Read the model definition and answer for the solid it produces. Units are mm, in the model's axes. A direction names the side the tool comes from. Coordinates: 2 decimals unless noted, no trailing zeros. Loops run counter-clockwise (first coordinate to the right, second up) from the corner with the lowest first, then second, coordinate; pieces in that order, holes last. Notation, with made-up numbers: (-27, 26.25) - (-9, 26.25) arc R35 ccw to (-9, 58.25) - close; hole circle Ø5 at (72.25, -33.75). An arc over 180 degrees is marked (long way). Use CSV: the item, a comma, the result in double quotes.
Autodesk Inventor part; units mm, degrees
ref_plane "Work Plane1" through (12.7, 70.5404, -12.7) normal (0, 0, -1) x (-1, 0, 0)
ref_plane "YZ Plane" through (0, 0, 0) normal (1, 0, 0) x (0, 1, 0)
ref_plane "XZ Plane" through (0, 0, 0) normal (0, 1, 0) x (-1, 0, 0)
sketch "Sketch1" plane through (0, 0, 0) normal (1, 0, 0) x (0, 1, 0)
  line L0 (0, 0) -> (76.2, 0)
  line L1 (76.2, 0) -> (76.2, -114.3)
  line L2 (76.2, -114.3) -> (0, -114.3)
  line L3 (0, -114.3) -> (0, 0)
  dimension "d0" = 76.2
  dimension "d1" = 114.3
extrude "Extrusion1" add sketch "Sketch1" along normal blind 12.7
sketch "Sketch2" plane through (12.7, 0, 0) normal (1, 0, 0) x (0, 0, -1)
  line L0 (0, 76.2) -> (0, 0)
  line L1 (0, 76.2) -> (25.4, 76.2)
  line L2 (25.4, 76.2) -> (25.4, 70.5404)
  line L3 (25.4, 70.5404) -> (0, 70.5404)
  line L4 (0, 70.5404) -> (0, 76.2)
  dimension "d4" = 25.4
extrude "Extrusion2" add sketch "Sketch2" along normal blind 12.7
sketch "Sketch3" plane through (0, 76.2, 0) normal (0, 1, 0) x (1, 0, 0)
  line L0 (0, 0) -> (0, 114.3)
  line L1 (0, 0) -> (25.4, 0)
  line L2 (25.4, 25.4) -> (25.4, 0)
  line L3 (12.7, 25.4) -> (25.4, 25.4)
  line L4 (12.7, 114.3) -> (12.7, 25.4)
  line L5 (0, 114.3) -> (12.7, 114.3)
  line L6 (12.7, 25.4) -> (25.4, 25.4)
  line L7 (22.225, 25.4) -> (22.225, 0)
  line L8 (0, 0) -> (25.4, 0)
  dimension "d8" = 3.175
extrude "Extrusion3" add sketch "Sketch3" along normal blind 25.4 contours L7 L3 L2 L1
sketch "Sketch4" plane through (0, 0, 0) normal (0, 0, 1) x (1, 0, 0)
  line L0 (0, 76.2) -> (22.225, 76.2)
  line L1 (0, 76.2) -> (22.225, 101.6)
  line L2 (22.225, 101.6) -> (19.8356, 103.6908)
  line L3 (19.8356, 103.6908) -> (0, 81.0215)
  line L4 (22.225, 101.6) -> (25.4, 101.6)
  line L5 (22.225, 76.2) -> (22.225, 101.6)
  line L6 (0, 76.2) -> (0, 81.0215)
  line L7 (22.225, 97.3812) -> (20.1342, 99.2106)
  line L8 (3.175, 76.2) -> (3.175, 79.8286)
  point P0 (0, 0)
  dimension "d11" = 3.175
  dimension "d12" = 3.175
  dimension "d13" = 3.175
extrude "Extrusion4" add sketch "Sketch4" against normal blind 3.175 contours L1 L8 L0 | L6 L3 L2 L1 | L1 L5 L7
ref_plane "Work Plane1" through (12.7, 70.5404, -12.7) normal (0, 0, -1) x (-1, 0, 0)
mirror "Mirror1" about plane through (12.7, 70.5404, -12.7) normal (0, 0, -1) of "Extrusion4"
sketch "Sketch5" plane through (25.4, 0, 0) normal (1, 0, 0) x (0, 0, -1)
  line L0 (0, 70.5404) -> (0, 101.6)
  line L1 (0, 70.5404) -> (25.4, 70.5404)
  line L2 (25.4, 70.5404) -> (25.4, 101.6)
  line L3 (0, 101.6) -> (25.4, 101.6)
  circle A0 centre (12.7, 88.9) radius 6.35
  line L4 (0, 76.2) -> (25.4, 76.2)
  circle A1 centre (12.7, 98.425) radius 1.778
  point P0 (0, 0)
  dimension "d16" = 12.7
  dimension "d17" = 25.4
  dimension "d18" = 25.4
  dimension "d19" = 12.7
  dimension "d20" = 12.7
  dimension "d21" = 3.556
  dimension "d22" = 9.525
extrude "Extrusion5" cut sketch "Sketch5" against normal blind 3.175 contours A1
pattern_circular "Circular Pattern1" count 8 over 360 about axis through (25.4, 88.9, -12.7) along (1, 0, 0) of "Extrusion5"
sketch "Sketch6" plane through (0, 0, 0) normal (-1, 0, 0) x (0, 0, 1)
  line L0 (0, 0) -> (-114.3, 0)
  line L1 (-20.0153, 0) -> (-20.0153, 59.8716) construction
  line L2 (-10.4903, 0) -> (-10.4903, 59.8716)
  line L3 (-29.5403, 59.8716) -> (-29.5403, 0)
  arc A0 (-29.5403, 0) -> (-10.4903, 0) centre (-20.0153, 0) ccw
  arc A1 (-10.4903, 59.8716) -> (-29.5403, 59.8716) centre (-20.0153, 59.8716) ccw
  line L4 (-20.0153, 59.8716) -> (-96.2153, 59.8716) construction
  line L5 (-20.0153, 69.3966) -> (-96.2153, 69.3966)
  line L6 (-96.2153, 50.3466) -> (-20.0153, 50.3466)
  arc A2 (-20.0153, 50.3466) -> (-20.0153, 69.3966) centre (-20.0153, 59.8716) ccw
  arc A3 (-96.2153, 69.3966) -> (-96.2153, 50.3466) centre (-96.2153, 59.8716) ccw
  line L7 (-96.2153, 59.8716) -> (-96.2153, 0) construction
  line L8 (-105.7403, 59.8716) -> (-105.7403, 0)
  line L9 (-86.6903, 0) -> (-86.6903, 59.8716)
  arc A4 (-86.6903, 59.8716) -> (-105.7403, 59.8716) centre (-96.2153, 59.8716) ccw
  arc A5 (-105.7403, 0) -> (-86.6903, 0) centre (-96.2153, 0) ccw
  line L10 (-114.3, 0) -> (-114.3, 76.2)
  line L11 (0, 0) -> (0, 81.0215)
  point P0 (-20.0153, 29.9358)
  point P1 (-58.1153, 59.8716)
  point P2 (-96.2153, 29.9358)
  dimension "d28" = 19.05
  dimension "d29" = 76.2
  dimension "d30" = 19.05
  dimension "d31" = 19.05
  dimension "d32" = 95.25
  dimension "d36" = 116.2307
  dimension "d37" = 10.4903
sketch "Sketch7" plane through (12.7, 0, 0) normal (1, 0, 0) x (0, 0, -1)
  line L0 (25.4, 70.5404) -> (0, 70.5404)
  line L1 (0, 70.5404) -> (0, 0)
  line L2 (0, 0) -> (114.3, 0) construction
  line L3 (114.3, 0) -> (114.3, 76.2)
  line L4 (114.3, 76.2) -> (25.4, 76.2)
  line L5 (25.4, 76.2) -> (25.4, 70.5404)
  line L6 (105.7403, 59.8716) -> (105.7403, 0)
  line L7 (20.0153, 69.3966) -> (96.2153, 69.3966)
  line L8 (0, 0) -> (0, 81.0215)
  line L9 (0, 81.0215) -> (3.175, 81.0215)
  line L10 (3.175, 76.2) -> (3.175, 81.0215)
  line L11 (3.175, 76.2) -> (22.225, 76.2)
  line L12 (22.225, 76.2) -> (22.225, 81.0215)
  line L13 (25.4, 81.0215) -> (22.225, 81.0215)
  line L14 (25.4, 81.0215) -> (25.4, 76.2)
  line L15 (25.4, 76.2) -> (114.3, 76.2)
  line L16 (114.3, 76.2) -> (114.3, 0)
  line L17 (114.3, 0) -> (0, 0)
  arc A0 (105.7403, 59.8716) -> (86.6903, 59.8716) centre (96.2153, 59.8716) ccw
  arc A1 (96.2153, 50.3466) -> (96.2153, 69.3966) centre (96.2153, 59.8716) ccw
  line L18 (96.2153, 50.3466) -> (20.0153, 50.3466)
  line L19 (86.6903, 0) -> (86.6903, 59.8716)
  arc A2 (86.6903, 0) -> (105.7403, 0) centre (96.2153, 0) ccw
  arc A3 (10.4903, 0) -> (29.5403, 0) centre (20.0153, 0) ccw
  line L20 (29.5403, 59.8716) -> (29.5403, 0)
  line L21 (10.4903, 0) -> (10.4903, 59.8716)
  arc A4 (29.5403, 59.8716) -> (10.4903, 59.8716) centre (20.0153, 59.8716) ccw
  arc A5 (20.0153, 69.3966) -> (20.0153, 50.3466) centre (20.0153, 59.8716) ccw
extrude "Extrusion7" cut sketch "Sketch7" against normal blind 11.43 contours L21 A5 L18 L20 L17 | L17 A3 | A4 L20 L18 A5 | L17 L19 L18 A1 L6 | A2 L17 | L20 A4 L7 A0 L19 L18 | A1 L18 L19 A0
fillet "Fillet2" radius 9.525 7 edges at (1.27, 66.6068, -102.9505) (1.27, 29.9358, -105.7403) (1.27, 29.9358, -10.4903) (1.27, 69.3966, -58.1153) (1.27, 25.1733, -86.6903) (1.27, 50.3466, -58.1153) (1.27, 25.1733, -29.5403)
equation "\"d12\" = d13"
equation "\"d19\" = 0.5 * d18"
equation "\"d20\" = 0.5 * d17"
equation "\"d28\" = d31"
equation "\"d30\" = d31"
equation "\"d37\" = -0.5 * d32 + 0.5 * d36"
properties part number "relicmold"
Q1. The part is cut by section D-D on z = -12.7. Give the number of separate pieces and of enclosed holes in the cut face, and give its area (3 significant figures).
Reported:
separate pieces,"3"
enclosed holes,"0"
area,"578 mm²"
Q2. A tool of negligible diameter and unlimited length cuts with its end or side. For faces 4 (the face through (23, 86, -25.4)), 5 (the face through (23.835, 90.596, -2.641)), 6 (the face through (11, 90, -22.225)), 7 (the face through (4.13, 30.35, -103.02)), 8 (the face through (19, 70.54, -13)), from which of +Z, -Z, +X, -X, +Y, -Y can it reach the whole face along a straight path? Write none if from no direction.
Reported:
face 4,"-Z, +X, +Y"
face 5,"+X"
face 6,"-X, +Y"
face 7,"+X, -Y"
face 8,"+Z, -Z, +X, -Y"
Q3. For a pull along X with two mould halves and no side action, classify faces 1 (the face through (23.835, 90.676, -22.303)), 2 (the face through (3.175, 78, -24)), 3 (the face through (12.7, 25, -58)) as +X half, -X half, draft (parallel to the pull), parting line (faces both ways), or undercut.
Reported:
face 1,"draft"
face 2,"undercut"
face 3,"+X half"
Q4. Given P1, Ø3, axis at x = 8.5, z = -22, coming from the +Y side; P2, Ø4.5, axis at y = 88.9, z = -3.175, coming from the -X side; P3, Ø12.5, axis at x = 8.5, y = 86.5, coming from the -Z side, each flat-ended and moving along its own axis, determine where each tip first touches the part or whether it passes through.
Reported:
P1,"stops at y = 92.43"
P2,"stops at x = 4.92"
P3,"stops at z = -25.4"
Q5. The part is cut by section B-B on y = 88.9. Determine the outline of the cut face in (x, z) (1 decimal).
Reported:
outline,"(6.9, -25.4) - (11.1, -25.4) - (11.1, -22.2) - (6.9, -22.2) - close; (6.9, -3.2) - (11.1, -3.2) - (11.1, 0) - (6.9, 0) - close; (22.2, -25.4) - (25.4, -25.4) - (25.4, -24) - (22.2, -24) - close; (22.2, -20.4) - (25.4, -20.4) - (25.4, -5) - (22.2, -5) - close; (22.2, -1.4) - (25.4, -1.4) - (25.4, 0) - (22.2, 0) - close"
Q6. Find the intervals of material crossed by probe 1 along Y at (x, z) = (23.6, -12.7); probe 2 along Z at (x, y) = (23.85, 88.9); probe 3 along Z at (x, y) = (13, 92.5) (3 decimals), in increasing order. Write a range as [from, to].
Reported:
probe 1,"y = [70.54, 77.6], [81.15, 96.65], [100.2, 101.6]"
probe 2,"z = [-25.4, -24], [-20.45, -4.95], [-1.4, 0]"
probe 3,"z = [-25.4, -22.225], [-3.175, 0]"
